Check sheet for the modelled part. Datum: model origin and axes. Units: mm. A direction names the side the tool comes from. Round coordinates to 2 decimals unless told otherwise and drop trailing zeros. Write each loop counter-clockwise with the first axis right and the second up, starting at its lowest first coordinate (ties: lowest second). Pieces come first, ordered by that corner, then holes.
from build123d import *

# Parameters (mm, degrees)
SKETCH1_W           = 42.1
SKETCH1_H           = 49
SKETCH1_W_2         = 39.1
SKETCH1_H_2         = 46
BOSS_EXTRUDE1_DEPTH = 8
SKETCH1_2_W         = 42.1
SKETCH1_2_H         = 49
BOSS_EXTRUDE2_DEPTH = 2.2
FILLET1_R           = 5
SKETCH2_W           = 3.4
SKETCH2_H           = 5.7
CUT_EXTRUDE1_DEPTH  = 1.5
FILLET2_R           = 1
SKETCH3_R           = 1.375
CUT_EXTRUDE2_DEPTH  = 2.2
SKETCH4_R           = 1.5
BOSS_EXTRUDE3_DEPTH = 0.2


with BuildPart() as part:
    # Sketch1 → Boss-Extrude1 (new body)
    with BuildSketch(Plane.XY):
        Rectangle(SKETCH1_W, SKETCH1_H)
        Rectangle(SKETCH1_W_2, SKETCH1_H_2, mode=Mode.SUBTRACT)
    extrude(amount=BOSS_EXTRUDE1_DEPTH)

    # Sketch1<2> → Boss-Extrude2 (add)
    with BuildSketch(Plane.XY):
        Rectangle(SKETCH1_2_W, SKETCH1_2_H)
    extrude(amount=-BOSS_EXTRUDE2_DEPTH)

    # Fillet1
    fillet1_edges = [part.edges().sort_by_distance(p)[0] for p in [
        (-19.55, 23, 4),
        (-19.55, -23, 4),
        (19.55, -23, 4),
        (19.55, 23, 4),
        (-21.05, 24.5, 2.9),
        (21.05, 24.5, 2.9),
        (21.05, -24.5, 2.9),
        (-21.05, -24.5, 2.9),
    ]]
    fillet(fillet1_edges, radius=FILLET1_R)

    # Sketch2 → Cut-Extrude1 (cut)
    with BuildSketch(Plane(origin=(0, 24.5, 0), x_dir=(1, 0, 0), z_dir=(0, 1, 0))):
        with Locations((0, -5.15)):
            Rectangle(SKETCH2_W, SKETCH2_H)
    extrude(amount=-CUT_EXTRUDE1_DEPTH, mode=Mode.SUBTRACT)

    # Fillet2
    fillet2_edges = [part.edges().sort_by_distance(p)[0] for p in [
        (1.7, 23.75, 8),
        (-1.7, 23.75, 8),
    ]]
    fillet(fillet2_edges, radius=FILLET2_R)

    # Sketch3 → Cut-Extrude2 (cut)
    with BuildSketch(Plane.XY):
        with Locations((0, 9.8)):
            Circle(SKETCH3_R)
        with Locations((-9.75, 0)):
            Circle(SKETCH3_R)
        with Locations((0, -9.8)):
            Circle(SKETCH3_R)
        with Locations((9.75, 0)):
            Circle(SKETCH3_R)
    extrude(amount=-CUT_EXTRUDE2_DEPTH, mode=Mode.SUBTRACT)

    # Sketch4 → Boss-Extrude3 (add)
    with BuildSketch(Plane.XY):
        with Locations((-9.75, 0)):
            Circle(SKETCH4_R)
        with Locations((0, 9.8)):
            Circle(SKETCH4_R)
        with Locations((9.75, 0)):
            Circle(SKETCH4_R)
        with Locations((0, -9.8)):
            Circle(SKETCH4_R)
    extrude(amount=-BOSS_EXTRUDE3_DEPTH)


solid = part.part
1. Sectioned sample at A-A, the plane z = -1.25. Enter the section's corners in (x, y) (3 decimals), plus the area to 3 significant figures.
2. Scan lines: line 1 along Y through (x, z) = (0, -1) (3 decimals); line 2 along X through (y, z) = (3, 0.5); line 3 along Y through (x, z) = (-6, 1). Record each from-to range of solid material in increasing order.
3. Go/stop test with flat-tipped pins: pin 1 (1.2 mm diameter, centred on x = 0, y = 23.5, fed in from +Z); pin 2 (0.8 mm diameter, centred on x = -10, y = 0.5, fed in from -Z); pin 3 (2 mm diameter, centred on x = 0, y = -9.8, fed in from +Z). Record where each tip stops, or that it passes through.
4. Set-up check for faces 1 (the cylindrical face through (-0.3, 8.46, -1.19)), 2 (the cylindrical face through (-2.001, 23.74, 7.715)), 3 (the flat face through (-19.55, 0, 4)), 4 (the cylindrical face through (19.62, -23, 2.97)): record each of +Z, -Z, +X, -X, +Y, -Y from which the full face is reachable in a straight line by a thin tool's end or side.
5. Sectioned sample at C-C, the plane y = 9.8. Enter the section's corners in (x, z) (3 decimals).
6. Release check for a two-part mould opening along Y. For faces 5 (the flat face through (0, 23, 2)), 6 (the cylindrical face through (-19.62, 23, 2.83)), 7 (the flat face through (21.05, 0, 3)) record: released by +Y, released by -Y, zero draft, split by the parting line, or undercut.
7. Sectioned sample at B-B, the plane x = 5. Enter the section's corners in (y, z).
8. Sectioned sample at D-D, the plane z = 6. Enter the section's corners in (x, y), plus the area to 3 significant figures.
Computed values:
1. outline: (-21.05, -19.5) arc R5 ccw to (-16.05, -24.5) - (16.05, -24.5) arc R5 ccw to (21.05, -19.5) - (21.05, 19.5) arc R5 ccw to (16.05, 24.5) - (-16.05, 24.5) arc R5 ccw to (-21.05, 19.5) - close; hole circle Ø2.75 at (-9.75, 0); hole circle Ø2.75 at (0, -9.8); hole circle Ø2.75 at (0, 9.8); hole circle Ø2.75 at (9.75, 0)
1. area: 2,020 mm2
2. line 1: y = -24.5 to -11.175, -8.425 to 8.425, 11.175 to 24.5
2. line 2: x = -21.05 to -19.55, 19.55 to 21.05
2. line 3: y = -24.5 to -23, 23 to 24.5
3. pin 1: stops at z = 2.3
3. pin 2: stops at z = -0.2
3. pin 3: stops at z = 0
4. face 1: -Z
4. face 2: +Z, +Y
4. face 3: +Z
4. face 4: +Z, -Z, +X, -Y
5. outline: (-21.05, -2.2) - (-1.375, -2.2) - (-1.375, -0.2) - (1.375, -0.2) - (1.375, -2.2) - (21.05, -2.2) - (21.05, 8) - (19.55, 8) - (19.55, 0) - (-19.55, 0) - (-19.55, 8) - (-21.05, 8) - close
6. face 5: undercut
6. face 6: released by +Y
6. face 7: zero draft
7. outline: (-24.5, -2.2) - (24.5, -2.2) - (24.5, 8) - (23, 8) - (23, 0) - (-23, 0) - (-23, 8) - (-24.5, 8) - close
8. outline: (-21.05, -19.5) arc R5 ccw to (-16.05, -24.5) - (16.05, -24.5) arc R5 ccw to (21.05, -19.5) - (21.05, 19.5) arc R5 ccw to (16.05, 24.5) - (1.7, 24.5) - (1.7, 23) - (14.55, 23) arc R5 cw to (19.55, 18) - (19.55, -18) arc R5 cw to (14.55, -23) - (-14.55, -23) arc R5 cw to (-19.55, -18) - (-19.55, 18) arc R5 cw to (-14.55, 23) - (-1.7, 23) - (-1.7, 24.5) - (-16.05, 24.5) arc R5 ccw to (-21.05, 19.5) - close
8. area: 259 mm2
